from build123d import *

# Parameters (mm, degrees)
F0_R     = 11.05
F1_DEPTH = 7
F3_DEPTH = 7
F4_DEPTH = 7


with BuildPart() as f1:
    # F0 (on Top) → F1 (new body)
    with BuildSketch(Plane.XY):
        with BuildLine():
            ThreePointArc((13.488193, 28.70727), (13.534539, 29.352897), (13.55, 30))
            ThreePointArc((13.55, 30), (13.20438, 33.040864), (12.185151, 35.9266))
            ThreePointArc((12.185151, 35.9266), (0, 43.55), (-12.185151, 35.9266))
            ThreePointArc((-12.185151, 35.9266), (-13.334535, 32.406796), (-13.488193, 28.70727))
            ThreePointArc((-13.488193, 28.70727), (-12.828695, 25.637996), (-11.480581, 22.802865))
            ThreePointArc((-11.480581, 22.802865), (0, 16.45), (11.480581, 22.802865))
            ThreePointArc((11.480581, 22.802865), (12.828695, 25.637996), (13.488193, 28.70727))
        make_face()
        with Locations((0, 30)):
            Circle(F0_R, mode=Mode.SUBTRACT)
        with BuildLine():
            ThreePointArc((12.185151, 35.9266), (13.20438, 33.040864), (13.55, 30))
            ThreePointArc((13.55, 30), (13.534539, 29.352897), (13.488193, 28.70727))
            ThreePointArc((13.488193, 28.70727), (28.157661, 14.60085), (31.234669, -5.516715))
            ThreePointArc((31.234669, -5.516715), (34.169815, -7.77393), (36.384345, -10.741415))
            ThreePointArc((36.384345, -10.741415), (33.678256, 17.463494), (12.185151, 35.9266))
        make_face()
        with BuildLine():
            ThreePointArc((-13.488193, 28.70727), (-13.334535, 32.406796), (-12.185151, 35.9266))
            ThreePointArc((-12.185151, 35.9266), (-32.955792, 18.791336), (-37.124024, -7.810595))
            ThreePointArc((-37.124024, -7.810595), (-34.680269, -5.028838), (-31.574733, -3.012468))
            ThreePointArc((-31.574733, -3.012468), (-27.553625, 15.711029), (-13.488193, 28.70727))
        make_face()
        with BuildLine():
            ThreePointArc((38.069481, -17.285689), (37.641436, -13.906813), (36.384345, -10.741415))
            ThreePointArc((36.384345, -10.741415), (34.169815, -7.77393), (31.234669, -5.516715))
            ThreePointArc((31.234669, -5.516715), (28.346106, -4.287249), (25.252139, -3.755511))
            ThreePointArc((25.252139, -3.755511), (13.444849, -9.478319), (12.022155, -22.522037))
            ThreePointArc((12.022155, -22.522037), (13.562584, -25.257446), (15.691155, -27.564948))
            ThreePointArc((15.691155, -27.564948), (18.803373, -29.57099), (22.342429, -30.659654))
            ThreePointArc((22.342429, -30.659654), (33.297392, -27.608033), (38.069481, -17.285689))
        make_face()
        with Locations((24.519481, -17.285689)):
            Circle(F0_R, mode=Mode.SUBTRACT)
        with BuildLine():
            ThreePointArc((-31.574733, -3.012468), (-34.680269, -5.028838), (-37.124024, -7.810595))
            ThreePointArc((-37.124024, -7.810595), (-37.478901, -22.179596), (-24.712464, -28.783549))
            ThreePointArc((-24.712464, -28.783549), (-21.097968, -27.9801), (-17.835919, -26.228204))
            ThreePointArc((-17.835919, -26.228204), (-15.530394, -24.097492), (-13.777076, -21.493407))
            ThreePointArc((-13.777076, -21.493407), (-12.650556, -18.476376), (-12.267842, -15.278711))
            ThreePointArc((-12.267842, -15.278711), (-16.114684, -5.820845), (-25.470975, -1.733152))
            ThreePointArc((-25.470975, -1.733152), (-28.597456, -2.016877), (-31.574733, -3.012468))
        make_face()
        with Locations((-25.817842, -15.278711)):
            Circle(F0_R, mode=Mode.SUBTRACT)
        with BuildLine():
            ThreePointArc((-17.835919, -26.228204), (-21.097968, -27.9801), (-24.712464, -28.783549))
            ThreePointArc((-24.712464, -28.783549), (-1.51136, -37.906653), (22.342429, -30.659654))
            ThreePointArc((22.342429, -30.659654), (18.803373, -29.57099), (15.691155, -27.564948))
            ThreePointArc((15.691155, -27.564948), (-1.263615, -31.692933), (-17.835919, -26.228204))
        make_face()
    extrude(amount=F1_DEPTH)

    # F2 (on Top) → F3 (join)
    with BuildSketch(Plane.XY):
        with BuildLine():
            ThreePointArc((22.186179, -6.487718), (23.344779, -6.274527), (24.522428, -6.243789))
            ThreePointArc((24.522428, -6.243789), (22.462795, 11.65149), (9.020363, 23.642493))
            ThreePointArc((9.020363, 23.642493), (8.320455, 22.700455), (7.494648, 21.866579))
            ThreePointArc((7.494648, 21.866579), (20.523874, 10.634266), (22.186179, -6.487718))
        make_face()
        with BuildLine():
            ThreePointArc((13.539374, -18.735057), (-0.928614, -23.096638), (-14.999749, -17.587624))
            ThreePointArc((-14.999749, -17.587624), (-15.236978, -18.747162), (-15.725852, -19.825034))
            ThreePointArc((-15.725852, -19.825034), (-1.000586, -25.28504), (14.110088, -21.005709))
            ThreePointArc((14.110088, -21.005709), (13.711284, -19.898897), (13.539374, -18.735057))
        make_face()
        with BuildLine():
            ThreePointArc((-22.652675, -4.60145), (-20.066421, 11.474134), (-7.523773, 21.856575))
            ThreePointArc((-7.523773, 21.856575), (-8.361476, 22.681537), (-9.059772, 23.627419))
            ThreePointArc((-9.059772, 23.627419), (-21.948573, 12.593433), (-24.970128, -4.102083))
            Line((-24.970128, -4.102083), (-22.652675, -4.60145))
        make_face()
    extrude(amount=F3_DEPTH)

    # F2 (on Top) → F4 (join)
    with BuildSketch(Plane.XY):
        with BuildLine():
            ThreePointArc((22.186179, -6.487718), (23.344779, -6.274527), (24.522428, -6.243789))
            ThreePointArc((24.522428, -6.243789), (22.462795, 11.65149), (9.020363, 23.642493))
            ThreePointArc((9.020363, 23.642493), (8.320455, 22.700455), (7.494648, 21.866579))
            ThreePointArc((7.494648, 21.866579), (20.523874, 10.634266), (22.186179, -6.487718))
        make_face()
        with BuildLine():
            ThreePointArc((13.539374, -18.735057), (-0.928614, -23.096638), (-14.999749, -17.587624))
            ThreePointArc((-14.999749, -17.587624), (-15.236978, -18.747162), (-15.725852, -19.825034))
            ThreePointArc((-15.725852, -19.825034), (-1.000586, -25.28504), (14.110088, -21.005709))
            ThreePointArc((14.110088, -21.005709), (13.711284, -19.898897), (13.539374, -18.735057))
        make_face()
        with BuildLine():
            ThreePointArc((-22.652675, -4.60145), (-20.066421, 11.474134), (-7.523773, 21.856575))
            ThreePointArc((-7.523773, 21.856575), (-8.361476, 22.681537), (-9.059772, 23.627419))
            ThreePointArc((-9.059772, 23.627419), (-21.948573, 12.593433), (-24.970128, -4.102083))
            Line((-24.970128, -4.102083), (-22.652675, -4.60145))
        make_face()
    extrude(amount=F4_DEPTH)


solid = f1.part
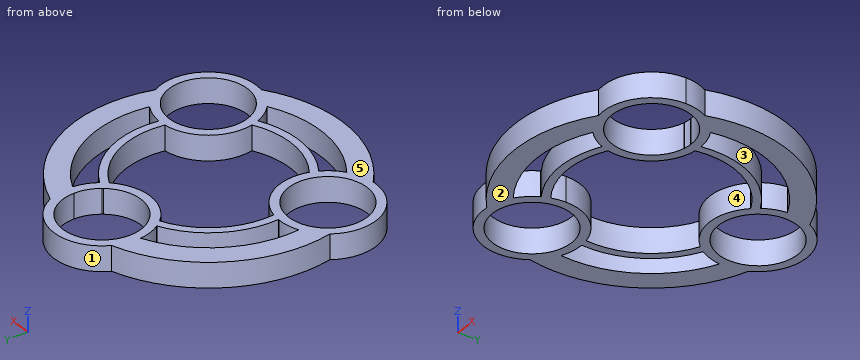
Can you work these out from the model? Positions are in its coordinate system, mm. Face numbers are marked on the shaded views. A direction names the side the tool comes from. Coordinates: 2 decimals unless noted, no trailing zeros. Loops run counter-clockwise (first coordinate to the right, second up) from the corner with the lowest first, then second, coordinate; pieces in that order, holes last. Notation, with made-up numbers: (-37.5, 20) - (9.5, 20) arc R28 cw to (9.5, 57) - close; hole circle Ø5 at (32, 33). An arc over 180 degrees is marked (long way). Put each result on its own line as item: value. Start each with the question number.
Item 1: Suppose I cut it at B-B (y = 6.5). Please give me the cut outline in (x, z), and give its area (3 significant figures).
Item 2: Suppose I cut it at C-C (z = 1.25). State how many separate pieces and enclosed holes the cut face has, and give its area (3 significant figures).
Item 3: If I drill on line 1 along Y through (x, z) = (-9.5, 1.5); line 2 along Y through (x, z) = (15, 6); line 3 along X through (y, z) = (8.5, 3.5), over which ranges is the centre line in solid material (lowest first)?
Item 4: If we mould it in two halves opening along Y, with no side actions, what happens to the marked faces 1, 2 and 3? For each: +Y half, -Y half, draft (parallel to the pull), parting line (faces both ways), or undercut.
Item 5: Suppose I cut it at A-A (x = 0). Please give me the cut outline in (y, z), and give its area (3 significant figures).
Item 6: Which directions (+Z, -Z, +X, -X, +Y, -Y) give clear straight access to the entire face, cutting with the end or side of a thin tool? Please do the marked faces 4 and 5.
Item 7: For pin 1 (4 mm diameter, centred on x = -27.5, z = 4.5, fed in from -Y); pin 2 (6 mm diameter, centred on x = 16, y = 8, fed in from -Z); pin 3 (2 mm diameter, centred on y = -9.5, z = 3.5, fed in from -X), each with a flat end and sliding along its axis, tell me the tip position at first contact or that it passes through.
Here are the results:
1. outline: (-37.38, 0) - (-31.04, 0) - (-31.04, 7) - (-37.38, 7) - close; (-24.46, 0) - (-22.18, 0) - (-22.18, 7) - (-24.46, 7) - close; (22.18, 0) - (24.46, 0) - (24.46, 7) - (22.18, 7) - close; (31.04, 0) - (37.38, 0) - (37.38, 7) - (31.04, 7) - close
1. area: 120 mm²
2. separate pieces: 1
2. enclosed holes: 7
2. area: 1,620 mm²
3. line 1: -36.73 to -30.26, -23.45 to -21.07, 20.34 to 24.36, 35.64 to 39.66
3. line 2: -34.85 to -27.95, -26.93 to -22.9, -11.67 to -7.64, 17.59 to 20.38, 27.95 to 34.85
3. line 3: -36.97 to -30.56, -23.83 to -21.5, 21.5 to 23.83, 30.56 to 36.97
4. face 1: +Y half
4. face 2: draft
4. face 3: undercut
5. outline: (-37.94, 0) - (-31.72, 0) - (-31.72, 7) - (-37.94, 7) - close; (-25.3, 0) - (-23.12, 0) - (-23.12, 7) - (-25.3, 7) - close; (16.45, 0) - (18.95, 0) - (18.95, 7) - (16.45, 7) - close; (41.05, 0) - (43.55, 0) - (43.55, 7) - (41.05, 7) - close
5. area: 93.9 mm²
6. face 4: +Z, -Z
6. face 5: +Z, +X, -X, +Y, -Y
7. pin 1: y = -28.83
7. pin 2: through
7. pin 3: x = -38.5
